Autodesk Inventor part; units mm, degrees
ref_plane "YZ Plane" through (0, 0, 0) normal (1, 0, 0) x (0, 1, 0)
ref_plane "XZ Plane" through (0, 0, 0) normal (0, 1, 0) x (-1, 0, 0)
ref_plane "XY Plane" through (0, 0, 0) normal (0, 0, 1) x (1, 0, 0)
sketch "草图1" plane through (0, 0, 0) normal (0, 1, 0) x (-1, 0, 0)
  line L0 (-20, 20) -> (20, 20)
  line L1 (20, 20) -> (20, -20)
  line L2 (20, -20) -> (-20, -20)
  line L3 (-20, -20) -> (-20, 20)
  line L4 (-20, 20) -> (20, -20) construction
  line L5 (20, 20) -> (-20, -20) construction
  line L6 (0, 40.4687) -> (0, -51.5947)
  line L7 (-15, -12) -> (15, -12) construction
  line L8 (15, -12) -> (15, 12) construction
  line L9 (15, 12) -> (-15, 12) construction
  line L10 (-15, 12) -> (-15, -12) construction
  line L11 (-15, -12) -> (15, 12) construction
  line L12 (15, -12) -> (-15, 12) construction
  circle A0 centre (15, 12) radius 1.75
  circle A1 centre (15, -12) radius 1.75
  circle A2 centre (-15, -12) radius 1.75
  circle A3 centre (-15, 12) radius 1.75
  point P0 (0, 0)
  point P1 (0, 0)
  dimension "d0" = 40
  dimension "d1" = 40
  dimension "d2" = 8
  dimension "d3" = 24
  dimension "d4" = 30
  dimension "d5" = 3.5
  dimension "d6" = 3.5
  dimension "d7" = 3.5
  dimension "d8" = 3.5
extrude "拉伸1" add sketch "草图1" along normal blind 1.5
sketch "草图3" plane through (20, 0, -20) normal (0, 0, -1) x (-1, 0, 0)
  line L0 (0, 0) -> (40, 0)
  line L1 (40, 0) -> (40, 27)
  line L2 (40, 47) -> (20, 47) construction
  line L3 (0, 27) -> (0, 0)
  line L4 (0, 0) -> (0, 1.5)
  line L5 (40, 0) -> (40, 1.5)
  arc A0 (40, 27) -> (0, 27) centre (20, 27) ccw
  line L6 (40, 27) -> (40, 47) construction
  line L7 (20, 20) -> (20, 34) construction
  line L8 (13.5, 20) -> (13.5, 34)
  line L9 (26.5, 34) -> (26.5, 20)
  arc A1 (13.5, 20) -> (26.5, 20) centre (20, 20) ccw
  arc A2 (26.5, 34) -> (13.5, 34) centre (20, 34) ccw
  circle A3 centre (20, 27) radius 15.5 construction
  circle A4 centre (4.5, 27) radius 1.6
  line L10 (20, 27) -> (4.5, 27) construction
  circle A5 centre (12.25, 13.5766) radius 1.6
  circle A6 centre (27.75, 13.5766) radius 1.6
  circle A7 centre (35.5, 27) radius 1.6
  circle A8 centre (27.75, 40.4234) radius 1.6
  circle A9 centre (12.25, 40.4234) radius 1.6
  point P0 (20, 0)
  dimension "d19" = 31
  dimension "d16" = 47
  dimension "d17" = 7
  dimension "d18" = 6.5
  dimension "d20" = 3.2
  dimension "d23" = 360
extrude "拉伸3" add sketch "草图3" against normal blind 1.5
fillet "圆角3" radius 3 1 edges at (0, 0, -20)
fillet "圆角4" radius 1.5 1 edges at (0, 1.5, -18.5)
properties part number "电机支架"
Build history of the part. All positions in model axes, mm. A direction names the side the tool comes from. Coordinates: 2 decimals unless noted, no trailing zeros. Order: outer loops, then holes, each group sorted by start corner. A loop starts at its lowest first (then second) coordinate and runs counter-clockwise, first axis right, second up.
Item 1: Saw through at D-D on x = 1.5. List the corners of the cut face in (y, z).
Filled in:
outline: (0, -17) arc R3 ccw to (3, -20) - (13.68, -20) - (13.68, -18.5) - (3, -18.5) arc R1.5 cw to (1.5, -17) - (1.5, 20) - (0, 20) - close; (40.32, -20) - (46.94, -20) - (46.94, -18.5) - (40.32, -18.5) - close
Item 2: Drill centre lines: L1, parallel to Y at x = 13, z = 16.5; L2, parallel to Z at x = 18, y = 20.5. Where is each one in solid material? Low to high.
Filled in:
L1: y = 0 to 1.5
L2: z = -20 to -18.5
Item 3: Drop flat-ended pins along their axis: pin 1 Ø3.5 at (x, y) = (15.5, 27) entering from +Z; pin 2 Ø0.8 at (y, z) = (30.5, -19.5) entering from -X; pin 3 Ø18.5 at (x, z) = (-1, 1) entering from +Y. Give the stop position or say it passes through.
Filled in:
pin 1: stops at z = -18.5
pin 2: stops at x = -19.76
pin 3: stops at y = 1.5
Item 4: Tool access for faces 1 (the flat face through (-9, 20, -18.5)), 2 (the cylindrical face through (-0.1, 40.5, -19.3)), 3 (the flat face through (0, 0, 2)): list every direction of +Z, -Z, +X, -X, +Y, -Y with a clear straight run to the whole face (end or side of a thin tool).
Filled in:
face 1: +Z, +X, -X, +Y
face 2: +Z, -Z
face 3: +Z, -Z, +X, -X, -Y
Item 5: Saw through at B-B on y = 22. List the corners of the cut face in (x, z), then the cut area to 3 significant figures.
Filled in:
outline: (-20, -20) - (-6.5, -20) - (-6.5, -18.5) - (-20, -18.5) - close; (6.5, -20) - (20, -20) - (20, -18.5) - (6.5, -18.5) - close
area: 40.5 mm2
Item 6: Saw through at C-C on x = -15.5. List the corners of the cut face in (y, z).
Filled in:
outline: (0, -17) arc R3 ccw to (3, -20) - (25.4, -20) - (25.4, -18.5) - (3, -18.5) arc R1.5 cw to (1.5, -17) - (1.5, -13.68) - (0, -13.68) - close; (0, -10.32) - (1.5, -10.32) - (1.5, 10.32) - (0, 10.32) - close; (0, 13.68) - (1.5, 13.68) - (1.5, 20) - (0, 20) - close; (28.6, -20) - (39.64, -20) - (39.64, -18.5) - (28.6, -18.5) - close
Item 7: Saw through at A-A on z = 12. List the corners of the cut face in (x, y), then the cut area to 3 significant figures.
Filled in:
outline: (-20, 0) - (-16.75, 0) - (-16.75, 1.5) - (-20, 1.5) - close; (-13.25, 0) - (13.25, 0) - (13.25, 1.5) - (-13.25, 1.5) - close; (16.75, 0) - (20, 0) - (20, 1.5) - (16.75, 1.5) - close
area: 49.5 mm2
Item 8: Mould opens along X. For faces 4 (the cylindrical face through (0, 47, -19)), 5 (the cylindrical face through (-16.669, 0.74, -12.526)), 6 (the flat face through (0, 1, 20)) say: released by +X, released by -X, zero draft, split by the parting line, or undercut.
Filled in:
face 4: split by the parting line
face 5: undercut
face 6: zero draft
